```python
from build123d import *

# Parameters (mm, degrees)
SKETCH025_W       = 50
SKETCH025_H       = 65
PAD015_DEPTH      = 10
SKETCH026_W       = 45
SKETCH026_H       = 30
POCKET008_DEPTH   = 10.001
SKETCH027_W       = 46
SKETCH027_H       = 60
POCKET009_DEPTH   = 8.001
SKETCH028_W       = 46
SKETCH028_H       = 100
POCKET010_DEPTH   = 5
CHAMFER002_SIZE   = 4
FILLET_R          = 1
CYLINDER004_R     = 4.5
CYLINDER004_DEPTH = 20
CYLINDER005_R     = 2.25
CYLINDER005_DEPTH = 20


with BuildPart() as part:
    # Sketch025 → Pad015 (new body)
    with BuildSketch(Plane.XY):
        Rectangle(SKETCH025_W, SKETCH025_H)
    extrude(amount=PAD015_DEPTH)

    # Sketch026 → Pocket008 (cut, through all)
    with BuildSketch(Plane.XY):
        Rectangle(SKETCH026_W, SKETCH026_H)
    extrude(amount=POCKET008_DEPTH, mode=Mode.SUBTRACT)

    # Sketch027 → Pocket009 (cut, through all)
    with BuildSketch(Plane.XY.offset(2)):
        Rectangle(SKETCH027_W, SKETCH027_H)
    extrude(amount=POCKET009_DEPTH, mode=Mode.SUBTRACT)

    # Sketch028 → Pocket010 (cut)
    with BuildSketch(Plane.XY.offset(6)):
        Rectangle(SKETCH028_W, SKETCH028_H)
    extrude(amount=POCKET010_DEPTH, mode=Mode.SUBTRACT)

    # Chamfer002
    chamfer002_edges = [part.edges().sort_by_distance(p)[0] for p in [
        (-24, -32.5, 10),
        (24, -32.5, 10),
        (24, 32.5, 10),
        (-24, 32.5, 10),
    ]]
    chamfer(chamfer002_edges, length=CHAMFER002_SIZE)

    # Fillet
    fillet_edges = [part.edges().sort_by_distance(p)[0] for p in [
        (25, 32.5, 3),
        (25, -32.5, 3),
        (-25, 32.5, 3),
        (-25, -32.5, 3),
    ]]
    fillet(fillet_edges, radius=FILLET_R)

    # Cylinder004 → Cylinder004 (join)
    with BuildSketch(Plane(origin=(0, 23, 0), x_dir=(1, 0, 0), z_dir=(0, 0, 1))):
        Circle(CYLINDER004_R)
    cylinder004 = extrude(amount=CYLINDER004_DEPTH)

    # Cylinder005 → Cylinder005 (cut)
    with BuildSketch(Plane(origin=(0, 23, 4), x_dir=(1, 0, 0), z_dir=(0, 0, 1))):
        Circle(CYLINDER005_R)
    cylinder005 = extrude(amount=CYLINDER005_DEPTH, mode=Mode.SUBTRACT)

    # Mirrored012: Cylinder004, Cylinder005 across XZ
    add(cylinder004.mirror(Plane.XZ))
    add(cylinder005.mirror(Plane.XZ), mode=Mode.SUBTRACT)


solid = part.part
```
Check sheet for the modelled part. Datum: model origin and axes. Units: mm. A direction names the side the tool comes from. Coordinates: 2 decimals unless noted, no trailing zeros. Order: outer loops, then holes, each group sorted by start corner. A loop starts at its lowest first (then second) coordinate and runs counter-clockwise, first axis right, second up. Notation, with made-up numbers: (81.25, 55.5) -> (133.25, 55.5) arc R14 cw to (133.25, 71.5) -> close; hole circle Ø5 at (6, 58). An arc over 180 degrees is marked (long way). Write each question's results on one line, items separated by ' | '. Start each with the question number.
1) Section check D-D (z = 8.75). Enter the section's corners in (x, y), and give its area (3 significant figures).
2) Section check B-B (x = 0). Enter the section's corners in (y, z).
3) Section check C-C (y = -0.5). Enter the section's corners in (x, z), and give its area (3 significant figures).
4) Depth check by flat-ended pin: pin 1 (2 mm diameter, centred on x = 4, y = -30.5, fed in from +Z); pin 2 (1 mm diameter, centred on x = -23.5, y = -12.5, fed in from +Z); pin 3 (2 mm diameter, centred on y = 21, z = 12.5, fed in from -X). Enter the tip coordinate at first touch or a pass-through.
5) Draft check along Y on faces 1 (the face through (-24, -30.5, 8)), 2 (the face through (-0.488, 20.804, 11.888)), 3 (the face through (24, 0, 10)). Enter one of: pulls with the +Y half, pulls with the -Y half, needs draft (parallel to the pull), parting line crosses it, or undercut.
6) Section check A-A (z = 5.25). Enter the section's corners in (x, y).
7) Set-up check for faces 4 (the face through (0, 15, 1)), 5 (the face through (-5, 20, 2)), 6 (the face through (-24, 0, 10)): record each of +Z, -Z, +X, -X, +Y, -Y from which the full face is reachable in a straight line by a thin tool's end or side.
8) Material ranges on line 1 along Y through (x, z) = (0, 8.75); line 2 along X through (y, z) = (23, 8); line 3 along Y through (x, z) = (0, 3), recorded low to high.
Checked values:
1) outline: (-25, -29.75) -> (-23, -29.75) -> (-23, 29.75) -> (-25, 29.75) -> close; circle Ø9 at (0, -23); circle Ø9 at (0, 23); (23, -29.75) -> (25, -29.75) -> (25, 29.75) -> (23, 29.75) -> close; hole circle Ø4.5 at (0, -23); hole circle Ø4.5 at (0, 23) | area: 333 mm²
2) outline: (-32.5, 0) -> (-15, 0) -> (-15, 2) -> (-18.5, 2) -> (-18.5, 20) -> (-20.75, 20) -> (-20.75, 4) -> (-25.25, 4) -> (-25.25, 20) -> (-27.5, 20) -> (-27.5, 2) -> (-30, 2) -> (-30, 6) -> (-32.5, 6) -> close; (15, 0) -> (32.5, 0) -> (32.5, 6) -> (30, 6) -> (30, 2) -> (27.5, 2) -> (27.5, 20) -> (25.25, 20) -> (25.25, 4) -> (20.75, 4) -> (20.75, 20) -> (18.5, 20) -> (18.5, 2) -> (15, 2) -> close
3) outline: (-25, 0) -> (-22.5, 0) -> (-22.5, 2) -> (-23, 2) -> (-23, 10) -> (-25, 10) -> close; (22.5, 0) -> (25, 0) -> (25, 10) -> (23, 10) -> (23, 2) -> (22.5, 2) -> close | area: 42.0 mm²
4) pin 1: z = 6 | pin 2: z = 10 | pin 3: x = -4.39
5) face 1: pulls with the -Y half | face 2: undercut | face 3: needs draft
6) outline: (-25, -31.5) arc R1 ccw to (-24, -32.5) -> (24, -32.5) arc R1 ccw to (25, -31.5) -> (25, 31.5) arc R1 ccw to (24, 32.5) -> (-24, 32.5) arc R1 ccw to (-25, 31.5) -> close; circle Ø9 at (0, -23); circle Ø9 at (0, 23); hole (-23, -30) -> (23, -30) -> (23, 30) -> (-23, 30) -> close; hole circle Ø4.5 at (0, -23); hole circle Ø4.5 at (0, 23)
7) face 4: +Z, -Z | face 5: +Z | face 6: +Z, -X, +Y, -Y
8) line 1: -27.5 to -25.25, -20.75 to -18.5, 18.5 to 20.75, 25.25 to 27.5 | line 2: -25 to -23, -4.5 to -2.25, 2.25 to 4.5, 23 to 25 | line 3: -32.5 to -30, -27.5 to -18.5, 18.5 to 27.5, 30 to 32.5
